```python
from build123d import *

# Parameters (mm, degrees)
SKETCH_1_W                = 40
SKETCH_1_H                = 20
EXTRUDE_1_DEPTH           = 149.5
SKETCH_2_W                = 38
SKETCH_2_H                = 18
CUT_EXTRUDE_1_DEPTH       = 149.5
SKETCH_4_R                = 1.525
CUT_EXTRUDE_2_DEPTH       = 10
SKETCH_5_R                = 1.525
CUT_EXTRUDE_3_DEPTH       = 21
SKETCH_6_R                = 1.525
CUT_EXTRUDE_4_DEPTH       = 21
SKETCH_7_R                = 1.525
CUT_EXTRUDE_5_DEPTH       = 1
CUT_EXTRUDE_5_DEPTH_BACK  = 41
CUT_EXTRUDE_START         = -21
SKETCH_9_R                = 2.025
CUT_EXTRUDE_6_DEPTH       = 22
CUT_EXTRUDE_7_DEPTH       = 1
CUT_EXTRUDE_7_DEPTH_BACK  = 21
SKETCH_11_R               = 4
CUT_EXTRUDE_8_DEPTH       = 22
SKETCH_12_R               = 1.525
CUT_EXTRUDE_9_DEPTH       = 1
CUT_EXTRUDE_9_DEPTH_BACK  = 21
SKETCH_13_R               = 1.525
CUT_EXTRUDE_10_DEPTH      = 1
CUT_EXTRUDE_10_DEPTH_BACK = 41


with BuildPart() as part:
    # 草图1 → 凸台-拉伸1 (new body, symmetric)
    with BuildSketch(Plane.XY):
        Rectangle(SKETCH_1_W, SKETCH_1_H)
    extrude(amount=EXTRUDE_1_DEPTH, both=True)

    # 草图2 → 切除-拉伸1 (cut, symmetric)
    with BuildSketch(Plane.XY):
        Rectangle(SKETCH_2_W, SKETCH_2_H)
    extrude(amount=CUT_EXTRUDE_1_DEPTH, both=True, mode=Mode.SUBTRACT)

    # 草图4 → 切除-拉伸2 (cut)
    with BuildSketch(Plane.ZY.offset(20)):
        with Locations((55, -6)):
            Circle(SKETCH_4_R)
        with Locations((55, 6)):
            Circle(SKETCH_4_R)
        with Locations((35, 6)):
            Circle(SKETCH_4_R)
        with Locations((35, -6)):
            Circle(SKETCH_4_R)
        with Locations((10, -6)):
            Circle(SKETCH_4_R)
        with Locations((10, 6)):
            Circle(SKETCH_4_R)
        with Locations((-10, 6)):
            Circle(SKETCH_4_R)
        with Locations((-10, -6)):
            Circle(SKETCH_4_R)
        with Locations((-35, 6)):
            Circle(SKETCH_4_R)
        with Locations((-55, -6)):
            Circle(SKETCH_4_R)
        with Locations((-55, 6)):
            Circle(SKETCH_4_R)
        with Locations((-35, -6)):
            Circle(SKETCH_4_R)
    extrude(amount=-CUT_EXTRUDE_2_DEPTH, mode=Mode.SUBTRACT)

    # 草图5 → 切除-拉伸3 (cut, through all)
    with BuildSketch(Plane.XZ.offset(10)):
        with Locations((-16, 65)):
            Circle(SKETCH_5_R)
        with Locations((-16, 45)):
            Circle(SKETCH_5_R)
        with Locations((-16, 20)):
            Circle(SKETCH_5_R)
        with Locations((-16, 0)):
            Circle(SKETCH_5_R)
        with Locations((-16, -45)):
            Circle(SKETCH_5_R)
        with Locations((-16, -65)):
            Circle(SKETCH_5_R)
    extrude(amount=-CUT_EXTRUDE_3_DEPTH, mode=Mode.SUBTRACT)

    # 草图6 → 切除-拉伸4 (cut, through all)
    with BuildSketch(Plane(origin=(0, 10, 0), x_dir=(1, 0, 0), z_dir=(0, 1, 0))):
        with Locations((-16, -81.75)):
            Circle(SKETCH_6_R)
        with Locations((-16, -101.75)):
            Circle(SKETCH_6_R)
    extrude(amount=-CUT_EXTRUDE_4_DEPTH, mode=Mode.SUBTRACT)

    # 草图7 → 切除-拉伸5 (cut, two sides)
    with BuildSketch(Plane.ZY.offset(20)) as cut_extrude_5_sk:
        with Locations((91.75, 6)):
            Circle(SKETCH_7_R)
        with Locations((111.75, 6)):
            Circle(SKETCH_7_R)
    extrude(amount=CUT_EXTRUDE_5_DEPTH, mode=Mode.SUBTRACT)
    extrude(cut_extrude_5_sk.sketch, amount=-CUT_EXTRUDE_5_DEPTH_BACK, mode=Mode.SUBTRACT)

    # 草图9 → 切除-拉伸6 (cut)
    with BuildSketch(Plane.XZ.offset(10).offset(CUT_EXTRUDE_START)):
        with Locations((14, -125.5)):
            Circle(SKETCH_9_R)
        with Locations((-14, -125.5)):
            Circle(SKETCH_9_R)
        with Locations((14, -143.5)):
            Circle(SKETCH_9_R)
        with Locations((-14, -143.5)):
            Circle(SKETCH_9_R)
    cut_extrude_6 = extrude(amount=CUT_EXTRUDE_6_DEPTH, mode=Mode.SUBTRACT)

    # 草图10 → 切除-拉伸7 (cut, two sides)
    with BuildSketch(Plane(origin=(0, 10, 0), x_dir=(1, 0, 0), z_dir=(0, 1, 0))) as cut_extrude_7_sk:
        with BuildLine():
            Line((-6, -89.5), (-6, -59.5))
            ThreePointArc((-6, -59.5), (0, -53.5), (6, -59.5))
            Line((6, -59.5), (6, -89.5))
            ThreePointArc((6, -89.5), (0, -95.5), (-6, -89.5))
        make_face()
        with BuildLine():
            Line((-6, 89.5), (-6, 59.5))
            ThreePointArc((-6, 59.5), (0, 53.5), (6, 59.5))
            Line((6, 59.5), (6, 89.5))
            ThreePointArc((6, 89.5), (0, 95.5), (-6, 89.5))
        make_face()
    extrude(amount=CUT_EXTRUDE_7_DEPTH, mode=Mode.SUBTRACT)
    extrude(cut_extrude_7_sk.sketch, amount=-CUT_EXTRUDE_7_DEPTH_BACK, mode=Mode.SUBTRACT)

    # 草图11 → 切除-拉伸8 (cut)
    with BuildSketch(Plane.XZ.offset(10).offset(CUT_EXTRUDE_START)):
        with Locations((0, -43)):
            Circle(SKETCH_11_R)
        with Locations((0, -106)):
            Circle(SKETCH_11_R)
    cut_extrude_8 = extrude(amount=CUT_EXTRUDE_8_DEPTH, mode=Mode.SUBTRACT)

    # 镜向1: 切除-拉伸8 across plane
    add(cut_extrude_8.mirror(Plane.XY), mode=Mode.SUBTRACT)

    # 镜向2: 切除-拉伸6 across plane
    add(cut_extrude_6.mirror(Plane.XY), mode=Mode.SUBTRACT)

    # 草图12 → 切除-拉伸9 (cut, two sides)
    with BuildSketch(Plane(origin=(0, 10, 0), x_dir=(1, 0, 0), z_dir=(0, 1, 0))) as cut_extrude_9_sk:
        with Locations((-16, 81.75)):
            Circle(SKETCH_12_R)
        with Locations((-16, 101.75)):
            Circle(SKETCH_12_R)
    extrude(amount=CUT_EXTRUDE_9_DEPTH, mode=Mode.SUBTRACT)
    extrude(cut_extrude_9_sk.sketch, amount=-CUT_EXTRUDE_9_DEPTH_BACK, mode=Mode.SUBTRACT)

    # 草图13 → 切除-拉伸10 (cut, two sides)
    with BuildSketch(Plane.ZY.offset(20)) as cut_extrude_10_sk:
        with Locations((-91.75, 6)):
            Circle(SKETCH_13_R)
        with Locations((-111.75, 6)):
            Circle(SKETCH_13_R)
    extrude(amount=CUT_EXTRUDE_10_DEPTH, mode=Mode.SUBTRACT)
    extrude(cut_extrude_10_sk.sketch, amount=-CUT_EXTRUDE_10_DEPTH_BACK, mode=Mode.SUBTRACT)


solid = part.part
```
Check sheet for the modelled part. Datum: model origin and axes. Units: mm. A direction names the side the tool comes from. Coordinates: 2 decimals unless noted, no trailing zeros. Loops run counter-clockwise (first coordinate to the right, second up) from the corner with the lowest first, then second, coordinate; pieces in that order, holes last. Notation, with made-up numbers: M 89.25,-14 L 103.25,-14 A38 cw 103.25,25 Z; hole C 9,22.5 d11. An arc over 180 degrees is marked long. Answer as a JSON object with one key per item and string values.
1. Depth check by flat-ended pin: P1, Ø1.8, axis at y = -6, z = 10, coming from the -X side. Enter the tip coordinate at first touch or a pass-through.
Outcome:
{"P1": "x = 19"}
2. Sectioned sample at A-A on z = 106. Record the cut outline in (x, y).
Outcome:
{"outline": "M -20,-10 L -4,-10 L -4,-9 L -19,-9 L -19,9 L -4,9 L -4,10 L -20,10 Z; M 4,-10 L 20,-10 L 20,10 L 4,10 L 4,9 L 19,9 L 19,-9 L 4,-9 Z"}
3. Sectioned sample at C-C on z = -120. Record the cut outline in (x, y).
Outcome:
{"outline": "M -20,-10 L 20,-10 L 20,10 L -20,10 Z; hole M -19,-9 L 19,-9 L 19,9 L -19,9 Z"}
4. Scan lines: L1, parallel to Z at x = 14, y = 9.6 (3 decimals); L2, parallel to X at y = -9.8, z = -81.75 (3 decimals); L3, parallel to Y at x = -2, z = 51.5. Record each from-to range of solid material in increasing order. Write a range as from..to.
Outcome:
{"L1": "-149.5..-145.525, -141.475..-127.525, -123.475..123.475, 127.525..141.475, 145.525..149.5", "L2": "-20..-17.525, -14.475..-6, 6..20", "L3": "-10..-9, 9..10"}
5. Sectioned sample at B-B on y = -0.75. Record the cut outline in (x, z), and give its area (3 significant figures).
Outcome:
{"outline": "M -20,-149.5 L -19,-149.5 L -19,149.5 L -20,149.5 Z; M 19,-149.5 L 20,-149.5 L 20,149.5 L 19,149.5 Z", "area": "598 mm²"}
6. Access from +Z, -Z, +X, -X, +Y, -Y to the whole of each face (thin tool, end or side, straight path). Record for faces 1 (the flat face through (0, 10, 2)), 2 (the flat face through (-19, 0, 2)), 3 (the cylindrical face through (-0.1, -9.5, -53.5)).
Outcome:
{"face 1": "+Z, -Z, +X, -X, +Y", "face 2": "+Z, -Z", "face 3": "+Y, -Y"}
7. Release check for a two-part mould opening along X. For faces 4 (the flat face through (20, 0, 2)), 5 (the flat face through (-20, 0, 2)), 6 (the flat face through (-1.6, -9.6, -149.5)), 7 (the cylindrical face through (0.1, -9.5, -95.5)) record: pulls with the +X half, pulls with the -X half, needs draft (parallel to the pull), parting line crosses it, or undercut.
Outcome:
{"face 4": "pulls with the +X half", "face 5": "pulls with the -X half", "face 6": "needs draft", "face 7": "undercut"}
